```python
from build123d import *

# Parameters (mm, degrees)
F0_R     = 3
F1_DEPTH = 300
F2_R     = 3.1
F3_DEPTH = 50
F4_R     = 3
F5_DEPTH = 50


with BuildPart() as f1:
    # F0 (on Right) → F1 (new body)
    with BuildSketch(Plane.YZ):
        Polygon((20, 7.5), (20, 20), (7.5, 20), (7.5, 12.5), (-7.5, 12.5), (-7.5, 20), (-20, 20), (-20, 7.5), (-12.5, 7.5), (-12.5, -7.5), (-20, -7.5), (-20, -20), (-7.5, -20), (-7.5, -12.5), (7.5, -12.5), (7.5, -20), (20, -20), (20, -7.5), (12.5, -7.5), (12.5, 7.5), align=None)
        Circle(F0_R, mode=Mode.SUBTRACT)
    extrude(amount=F1_DEPTH)

    # F2 (on face) → F3 (cut)
    with BuildSketch(Plane.XY.offset(12.5)):
        with Locations((250, 0)):
            Circle(F2_R)
        with Locations((211.5, 0)):
            Circle(F2_R)
    extrude(amount=-F3_DEPTH, mode=Mode.SUBTRACT)

    # F4 (on face) → F5 (cut)
    with BuildSketch(Plane.XY.offset(12.5)):
        with Locations((50, 0)):
            Circle(F4_R)
        with Locations((100, 0)):
            Circle(F4_R)
    extrude(amount=-F5_DEPTH, mode=Mode.SUBTRACT)


solid = f1.part
```
Input: part model. Units: mm. Frame: model coordinates. A direction names the side the tool comes from. Coordinates: 2 decimals unless noted, no trailing zeros. Write each loop counter-clockwise with the first axis right and the second up, starting at its lowest first coordinate (ties: lowest second). Pieces come first, ordered by that corner, then holes.
1) Material intervals for line 1 along X through (y, z) = (0, 5); line 2 along Y through (x, z) = (100, -8.25); line 3 along Y through (x, z) = (211, -4), sorted ascending.
2) Section A-A on x = 281.5. Output: boundary loops of the cut face in (y, z).
3) Mould query, pull axis Y, two halves, no side actions, for faces 5 (the cylindrical face through (51.61, 2.53, -7.55)), 6 (the flat face through (148, -16, 7.5)), 7 (the flat face through (148, 20, -14)). Classes: pulls with the +Y half, pulls with the -Y half, needs draft (parallel to the pull), parting line crosses it, or undercut.
4) Pin query (flat end, axial travel): pin 1 Ø3.5 at (x, y) = (100, 0) entering from +Z; pin 2 Ø7 at (x, y) = (211.5, 0) entering from +Z; pin 3 Ø7.5 at (x, z) = (216, 0) entering from -Y; pin 4 Ø7.5 at (x, z) = (114, -2.5) entering from +Y. Return the tip coordinate at first contact, or that it passes through.
5) Section B-B on y = 0. State how many separate pieces and enclosed holes the cut face has, and give its area (3 significant figures).
6) Set-up query: faces 1 (the flat face through (148, 0, 12.5)), 2 (the flat face through (148, 0, -12.5)), 3 (the flat face through (148, -16, -7.5)), 4 (the flat face through (148, 12.5, 0)). Return all of +Z, -Z, +X, -X, +Y, -Y with unobstructed straight access to the full face (end or side cutting, diameter ignored); none if empty.
Check result:
1. line 1: x = 0 to 47, 53 to 97, 103 to 208.4, 214.6 to 246.9, 253.1 to 300
1. line 2: y = -20 to -3, 3 to 20
1. line 3: y = -12.5 to -3.06, 3.06 to 12.5
2. outline: (-20, -20) - (-7.5, -20) - (-7.5, -12.5) - (7.5, -12.5) - (7.5, -20) - (20, -20) - (20, -7.5) - (12.5, -7.5) - (12.5, 7.5) - (20, 7.5) - (20, 20) - (7.5, 20) - (7.5, 12.5) - (-7.5, 12.5) - (-7.5, 20) - (-20, 20) - (-20, 7.5) - (-12.5, 7.5) - (-12.5, -7.5) - (-20, -7.5) - close; hole circle Ø6 at (0, 0)
3. face 5: undercut
3. face 6: needs draft
3. face 7: pulls with the +Y half
4. pin 1: passes through
4. pin 2: stops at z = 12.5
4. pin 3: stops at y = -12.5
4. pin 4: stops at y = 12.5
5. separate pieces: 10
5. enclosed holes: 0
5. area: 5,240 mm2
6. face 1: +Z, +X, -X
6. face 2: -Z, +X, -X
6. face 3: +X, -X, -Y
6. face 4: +X, -X, +Y
